from build123d import *

# Parameters (mm, degrees)
BOSS_EXTRUDE1_DEPTH = 25.4
FILLET1_R           = 1.5875
FILLET3_R           = 6.35
SKETCH2_R           = 2.5527
CUT_EXTRUDE1_DEPTH  = 47.797604439
SKETCH4_R           = 2.5527
CUT_EXTRUDE2_DEPTH  = 47.797604439


with BuildPart() as part:
    # Sketch1 → Boss-Extrude1 (new body)
    with BuildSketch(Plane.XY):
        Polygon((-5.3975, 26.9875), (5.3975, 26.9875), (14.2875, 18.0975), (14.2875, 6.35), (28.575, 6.35), (28.575, 0), (-28.575, 0), (-28.575, 6.35), (-14.2875, 6.35), (-14.2875, 18.0975), align=None)
    extrude(amount=-BOSS_EXTRUDE1_DEPTH)

    # Fillet1
    fillet1_edges = [part.edges().sort_by_distance(p)[0] for p in [
        (14.2875, 6.35, -12.7),
        (28.575, 6.35, -12.7),
        (-28.575, 6.35, -12.7),
        (-14.2875, 6.35, -12.7),
    ]]
    fillet(fillet1_edges, radius=FILLET1_R)

    # Fillet3
    fillet3_edges = [part.edges().sort_by_distance(p)[0] for p in [
        (-5.3975, 26.9875, -12.7),
        (5.3975, 26.9875, -12.7),
        (14.2875, 18.0975, -12.7),
        (-14.2875, 18.0975, -12.7),
    ]]
    fillet(fillet3_edges, radius=FILLET3_R)

    # Sketch2 → Cut-Extrude1 (cut, through all)
    with BuildSketch(Plane.XZ):
        with Locations(Location((-22.225, -12.7, 0), (0, 0, 180))):
            Circle(SKETCH2_R)
    cut_extrude1 = extrude(amount=-CUT_EXTRUDE1_DEPTH, mode=Mode.SUBTRACT)

    # Mirror1: Cut-Extrude1 across plane
    add(cut_extrude1.mirror(Plane(origin=(0, 0, 0), x_dir=(0, 0, 1), z_dir=(1, 0, 0))), mode=Mode.SUBTRACT)

    # Sketch4 → Cut-Extrude2 (cut, through all)
    with BuildSketch(Plane(origin=(0, 0, -25.4), x_dir=(-1, 0, 0), z_dir=(0, 0, -1))):
        with Locations(Location((0, 13.7668, 0), (0, 0, 180))):
            Circle(SKETCH4_R)
    extrude(amount=-CUT_EXTRUDE2_DEPTH, mode=Mode.SUBTRACT)


solid = part.part
CAD build for the part. Positions are in the model's coordinates, mm. A direction names the side the tool comes from. Coordinates: 2 decimals unless noted, no trailing zeros. Loops run counter-clockwise (first coordinate to the right, second up) from the corner with the lowest first, then second, coordinate; pieces in that order, holes last. Notation, with made-up numbers: (72, -10.5) -> (102, -10.5) arc R21 cw to (102, 28.5) -> close; hole circle Ø2 at (69, -30.5). An arc over 180 degrees is marked (long way). One line per item, written item: value.
1. Drill centre lines: line 1 (X direction, y = 4.5, z = -12.7) (3 decimals); line 2 (Y direction, x = 0, z = -13.5); line 3 (Z direction, x = 20, y = 3.25). Where is each one in solid material? Low to high. Write a range as [from, to].
Answers:
line 1: x = [-28.575, -24.778], [-19.672, 19.672], [24.778, 28.575]
line 2: y = [0, 11.21], [16.32, 26.99]
line 3: z = [-25.4, -13.95], [-11.45, 0]
2. Slice it at C-C on y = 3.25. Write the cut outline in (x, z) (3 decimals), and give its area (3 significant figures).
Answers:
outline: (-28.575, -25.4) -> (28.575, -25.4) -> (28.575, 0) -> (-28.575, 0) -> close; hole circle Ø5.105 at (-22.225, -12.7); hole circle Ø5.105 at (22.225, -12.7)
area: 1,410 mm^2
3. Slice it at A-A on x = 0. Write the cut outline in (y, z).
Answers:
outline: (0, -25.4) -> (11.21, -25.4) -> (11.21, 0) -> (0, 0) -> close; (16.32, -25.4) -> (26.99, -25.4) -> (26.99, 0) -> (16.32, 0) -> close
4. Slice it at B-B on z = -13.75. Give the number of separate pieces and of enclosed holes in the cut face, and give its area (3 significant figures).
Answers:
separate pieces: 3
enclosed holes: 1
area: 791 mm^2
5. Which spindle directions (+Z, -Z, +X, -X, +Y, -Y) get a long thin tool onto all of the face, cutting with end or side? Do faces 1 (the face through (19, 6.35, -13)), 2 (the face through (0, 11, 0)), 3 (the face through (-19, 6.35, -13)). Say none if no direction does.
Answers:
face 1: +Z, -Z, +X, +Y
face 2: +Z, +X, -X, +Y, -Y
face 3: +Z, -Z, -X, +Y
6. Flat gauge pins, fed straight in: P1, Ø12, axis at x = -20.5, z = -18.5, coming from the +Y side; P2, Ø6, axis at y = 8.5, z = -9, coming from the +X side; P3, Ø9, axis at x = 21, z = -11.5, coming from the +Y side; P4, Ø3, axis at x = 22.225, z = -12.7, coming from the +Y side. Where does each tip first touch, or does it go through?
Answers:
P1: stops at y = 7.14
P2: stops at x = 28.39
P3: stops at y = 6.35
P4: passes through
7. Pull direction Y, two halves, no side cores. Call faces 4 (the face through (-28.122, 5.873, -12.878)), 5 (the face through (-2.026, 15.32, -12.878)), 6 (the face through (28.575, 2, -13)): pulls with the +Y half, pulls with the -Y half, needs draft (parallel to the pull), parting line crosses it, or undercut.
Answers:
face 4: pulls with the +Y half
face 5: undercut
face 6: needs draft
